Here's how the part is built. I have some questions about the finished solid (model axes, mm). Round coordinates to 2 decimals unless told otherwise and drop trailing zeros. Write each loop counter-clockwise with the first axis right and the second up, starting at its lowest first coordinate (ties: lowest second). Pieces come first, ordered by that corner, then holes. Notation, with made-up numbers: M -24,60 L 23,60 A31 cw 23,97 Z; hole C 23,42.5 d11. An arc over 180 degrees is marked long. Use a Markdown table: item, result. Add a question column.
```python
from build123d import *
from build123d import SkipClean  # not in build123d's __all__

# Parameters (mm, degrees)
F1_DEPTH = 20
F2_R     = 16
F2_R_2   = 11
F3_DEPTH = 7


with BuildPart() as f1:
    # F0 (on Front) → F1 (new body)
    with BuildSketch(Plane.XZ):
        with BuildLine():
            Line((-2, 0), (0, 0))
            Line((0, 0), (10, 0))
            Line((10, 0), (12, 0))
            ThreePointArc((12, 0), (5, 7), (-2, 0))
        make_face()
    extrude(amount=F1_DEPTH)

    # F2 (on Top) → F3 (join)
    with BuildSketch(Plane.XY):
        with Locations((5, 11)):
            Circle(F2_R)
        with Locations((5, 11)):
            Circle(F2_R_2, mode=Mode.SUBTRACT)
    with SkipClean():  # cleaning this boolean's faces spoils the solid; the shape is the same uncleaned
        extrude(amount=F3_DEPTH)


solid = f1.part
```
Item 1: Imagine slicing it at A-A on y = 21.5. List the corners of the cut face in (x, z) for me, plus the area to 3 significant figures.
Item 2: If we mould it in two halves opening along X, with no side actions, what happens to faces 1 (the face through (2.62, 0.26, 3.45)), 2 (the face through (5, -1, 0)), 3 (the face through (5, -12, 7))? For each: +X half, -X half, draft (parallel to the pull), parting line (faces both ways), or undercut.
Item 3: Imagine slicing it at B-B on x = 11. List the corners of the cut face in (y, z) for me.
Item 4: Imagine slicing it at D-D on x = 4. List the corners of the cut face in (y, z) for me, plus the area to 3 significant figures.
Item 5: I need wall thicknesses on probe 1 along Y at (x, z) = (5, 2.25); probe 2 along X at (y, z) = (11, 1.5); probe 3 along X at (y, z) = (12.5, 1.75). Which ranges of each line are inside material? Lowest first, please. Write a range as from..to.
Item 6: Imagine slicing it at C-C on z = 4.5. List the corners of the cut face in (x, y) for me, plus the area to 3 significant figures.
Item 7: For pin 1 Ø1.5 at (x, y) = (5.5, 2.5) entering from -Z; pin 2 Ø1.5 at (y, z) = (13, 5) entering from +X; pin 3 Ø3 at (x, z) = (14.5, 6.5) entering from +Y; pin 4 Ø4 at (x, z) = (-6.5, 1.5) entering from +Y, each with a flat end and sliding along its axis, tell me the tip position at first contact or that it passes through.
The answers:
| question | item | result |
|---|---|---|
| 1 | outline | M -7.07,0 L 1.72,0 L 1.72,7 L -7.07,7 Z; M 8.28,0 L 17.07,0 L 17.07,7 L 8.28,7 Z |
| 1 | area | 123 mm² |
| 2 | face 1 | undercut |
| 2 | face 2 | draft |
| 2 | face 3 | parting line |
| 3 | outline | M -20,0 L 1.78,0 L 1.78,7 L -3.83,7 L -3.83,3.61 L -20,3.61 Z; M 20.22,0 L 25.83,0 L 25.83,7 L 20.22,7 Z |
| 4 | outline | M -20,0 L 0.05,0 L 0.05,7 L -4.97,7 L -4.97,6.93 L -20,6.93 Z; M 21.95,0 L 26.97,0 L 26.97,7 L 21.95,7 Z |
| 4 | area | 174 mm² |
| 5 | probe 1 | -20..0, 22..27 |
| 5 | probe 2 | -11..-6, 16..21 |
| 5 | probe 3 | -10.93..-5.9, 15.9..20.93 |
| 6 | outline | M -0.36,-20 L 10.36,-20 L 10.36,-4.07 A16 ccw long -0.36,-4.07 Z; hole C 5,11 d22 |
| 6 | area | 588 mm² |
| 7 | pin 1 | through |
| 7 | pin 2 | x = 20.95 |
| 7 | pin 3 | y = 24.86 |
| 7 | pin 4 | y = 23.87 |
